Read the model definition and answer for the solid it produces. Units are mm, in the model's axes. A direction names the side the tool comes from. Give positions to 0.01 mm unless a question says otherwise; leave off trailing zeros. Loops run counter-clockwise (first coordinate to the right, second up) from the corner with the lowest first, then second, coordinate; pieces in that order, holes last. Notation, with made-up numbers: (-13.5, 3) -> (41.5, 3) arc R23 ccw to (41.5, 37) -> close; hole circle Ø4 at (8, 15). An arc over 180 degrees is marked (long way). One line per item, written item: value. Start each with the question number.
from build123d import *

# Parameters (mm, degrees)
SCHIZZO2_R                   = 30
ESTRUSIONE_ESTRUSIONE1_DEPTH = 7.5
SCHIZZO3_W                   = 10
SCHIZZO3_H                   = 10
TAGLIO_ESTRUSIONE1_DEPTH     = 44.084219849
TAGLIO_ESTRUSIONE2_DEPTH     = 44.084219849


with BuildPart() as part:
    # Schizzo2 → Estrusione-Estrusione1 (new body)
    with BuildSketch(Plane.XY):
        Circle(SCHIZZO2_R)
    extrude(amount=ESTRUSIONE_ESTRUSIONE1_DEPTH)

    # Schizzo3 → Taglio-Estrusione1 (cut, through all)
    with BuildSketch(Plane(origin=(0, 0, 0), x_dir=(-1, 0, 0), z_dir=(0, 0, -1))):
        Rectangle(SCHIZZO3_W, SCHIZZO3_H)
    extrude(amount=-TAGLIO_ESTRUSIONE1_DEPTH, mode=Mode.SUBTRACT)

    # Schizzo4 → Taglio-Estrusione2 (cut, through all)
    with BuildSketch(Plane(origin=(0, 0, 0), x_dir=(-1, 0, 0), z_dir=(0, 0, -1))):
        with BuildLine():
            Line((-0.285302534, 29.998643344), (-0.89, 22.45))
            Line((-0.89, 22.45), (13.755471769, 26.660588823))
            ThreePointArc((13.755471769, 26.660588823), (6.938805142, 29.186520574), (-0.285302534, 29.998643344))
        make_face()
        with BuildLine():
            Line((10.454237391, 19.887270315), (25.242882405, 16.211011316))
            ThreePointArc((25.242882405, 16.211011316), (20.602441812, 21.806865694), (14.75224243, 26.122238482))
            Line((14.75224243, 26.122238482), (10.454237391, 19.887270315))
        make_face()
        with BuildLine():
            Line((18.997270315, 11.995762609), (29.966483085, 1.417706418))
            ThreePointArc((29.966483085, 1.417706418), (28.745670836, 8.584078762), (25.836935948, 15.246400914))
            Line((25.836935948, 15.246400914), (18.997270315, 11.995762609))
        make_face()
        with BuildLine():
            Line((22.45, 0.89), (26.660588823, -13.755471769))
            ThreePointArc((26.660588823, -13.755471769), (29.186520574, -6.938805142), (29.998643344, 0.285302534))
            Line((29.998643344, 0.285302534), (22.45, 0.89))
        make_face()
        with BuildLine():
            Line((19.887270315, -10.454237391), (16.211011316, -25.242882405))
            ThreePointArc((16.211011316, -25.242882405), (21.806865694, -20.602441812), (26.122238482, -14.75224243))
            Line((26.122238482, -14.75224243), (19.887270315, -10.454237391))
        make_face()
        with BuildLine():
            Line((11.995762609, -18.997270315), (1.417706418, -29.966483085))
            ThreePointArc((1.417706418, -29.966483085), (8.584078762, -28.745670836), (15.246400914, -25.836935948))
            Line((15.246400914, -25.836935948), (11.995762609, -18.997270315))
        make_face()
        with BuildLine():
            Line((0.89, -22.45), (-13.755471769, -26.660588823))
            ThreePointArc((-13.755471769, -26.660588823), (-6.938805142, -29.186520574), (0.285302534, -29.998643344))
            Line((0.285302534, -29.998643344), (0.89, -22.45))
        make_face()
        with BuildLine():
            Line((-10.454237391, -19.887270315), (-25.242882405, -16.211011316))
            ThreePointArc((-25.242882405, -16.211011316), (-20.602441812, -21.806865694), (-14.75224243, -26.122238482))
            Line((-14.75224243, -26.122238482), (-10.454237391, -19.887270315))
        make_face()
        with BuildLine():
            Line((-18.997270315, -11.995762609), (-29.966483085, -1.417706418))
            ThreePointArc((-29.966483085, -1.417706418), (-28.745670836, -8.584078762), (-25.836935948, -15.246400914))
            Line((-25.836935948, -15.246400914), (-18.997270315, -11.995762609))
        make_face()
        with BuildLine():
            Line((-22.45, -0.89), (-26.660588823, 13.755471769))
            ThreePointArc((-26.660588823, 13.755471769), (-29.186520574, 6.938805142), (-29.998643344, -0.285302534))
            Line((-29.998643344, -0.285302534), (-22.45, -0.89))
        make_face()
        with BuildLine():
            Line((-19.887270315, 10.454237391), (-16.211011316, 25.242882405))
            ThreePointArc((-16.211011316, 25.242882405), (-21.806865694, 20.602441812), (-26.122238482, 14.75224243))
            Line((-26.122238482, 14.75224243), (-19.887270315, 10.454237391))
        make_face()
        with BuildLine():
            Line((-11.995762609, 18.997270315), (-1.417706418, 29.966483085))
            ThreePointArc((-1.417706418, 29.966483085), (-8.584078762, 28.745670836), (-15.246400914, 25.836935948))
            Line((-15.246400914, 25.836935948), (-11.995762609, 18.997270315))
        make_face()
    extrude(amount=-TAGLIO_ESTRUSIONE2_DEPTH, mode=Mode.SUBTRACT)


solid = part.part
Item 1: Section A-A, the plane x = -24 is taken. Determine the outline of the cut face in (y, z), plus the area to 3 significant figures.
Item 2: Determine the mould class of faces 4 (the flat face through (12.6, -23, 3.7)), 5 (the flat face through (6, 0, 0)), 6 (the flat face through (13.64, 22.46, 3.7)) for opening direction X: pulls with the +X half, pulls with the -X half, needs draft (parallel to the pull), parting line crosses it, or undercut.
Item 3: Section C-C, the plane x = 3 is taken. Determine the outline of the cut face in (y, z), plus the area to 3 significant figures.
Item 4: Section B-B, the plane y = 21 is taken. Determine the outline of the cut face in (x, z).
Item 5: Flat-ended cylindrical pins translate along their axes: pin 1 (1.5 mm diameter, centred on y = 6.5, z = 5, fed in from +X); pin 2 (3 mm diameter, centred on x = 20.5, z = 2, fed in from -Y); pin 3 (2 mm diameter, centred on y = 1, z = 3.5, fed in from +X). Find the tip coordinate at first contact, or state that the pin passes through.
Item 6: Consider L1, parallel to X at y = -13.5, z = 5.75; L2, parallel to Y at x = 4, z = 5.5; L3, parallel to X at y = -2, z = 6. Determine where each line is inside the solid, lowest interval first. Write a range as [from, to].
Item 7: For faces 1 (the flat face through (-17.745, 18.075, 3.698)), 2 (the flat face through (0.583, 26.277, 3.698)), 3 (the flat face through (-6.781, -24.405, 3.698)), determine the directions among +Z, -Z, +X, -X, +Y, -Y from which every point of the face is accessible in a straight line to the end or side of a thin tool.
Computed values:
1. outline: (-13.29, 0) -> (-4.5, 0) -> (-4.5, 7.5) -> (-13.29, 7.5) -> close; (0.77, 0) -> (7.17, 0) -> (7.17, 7.5) -> (0.77, 7.5) -> close; (14.37, 0) -> (16.52, 0) -> (16.52, 7.5) -> (14.37, 7.5) -> close
1. area: 130 mm²
2. face 4: pulls with the +X half
2. face 5: needs draft
2. face 6: undercut
3. outline: (-23.57, 0) -> (-5, 0) -> (-5, 7.5) -> (-23.57, 7.5) -> close; (5, 0) -> (28.33, 0) -> (28.33, 7.5) -> (5, 7.5) -> close
3. area: 314 mm²
4. outline: (-11.22, 0) -> (10.06, 0) -> (10.06, 7.5) -> (-11.22, 7.5) -> close; (12.95, 0) -> (17.27, 0) -> (17.27, 7.5) -> (12.95, 7.5) -> close
5. pin 1: x = 24.79
5. pin 2: y = -17.76
5. pin 3: x = 23.28
6. L1: [-26.59, -24.31], [-19.13, 22.16]
6. L2: [-23.86, -5], [5, 27.29]
6. L3: [-23.28, -5], [5, 29.36]
7. face 1: +Z, -Z, -X
7. face 2: +Z, -Z
7. face 3: +Z, -Z, -Y
